Design review of the part built by this model. Coordinates are the model's own, in mm. A direction names the side the tool comes from. Round coordinates to 2 decimals unless told otherwise and drop trailing zeros. Loops run counter-clockwise (first coordinate to the right, second up) from the corner with the lowest first, then second, coordinate; pieces in that order, holes last. Notation, with made-up numbers: (42, -13.5) - (86, -13.5) arc R23 ccw to (86, 21.5) - close; hole circle Ø2 at (-6.75, 42.5). An arc over 180 degrees is marked (long way). Answer as CSV lines item,"result". Start each with the question number.
(1) Consider section A-A (y = -20). Give the boundary of the cut face in (x, z), and give its area (3 significant figures).
(2) For faces 4 (the cylindrical face through (-26.09, -81.57, -22.99)), 5 (the cylindrical face through (-23.92, 5.83, 27.37)), 6 (the flat face through (-23, 0, 22)), 7 (the flat face through (28, 6, -28)), list the 3-axis set-ups (+Z, -Z, +X, -X, +Y, -Y) from which the entire face can be reached by the end or side of a thin tool; tool diameter is ignored.
(3) For P1, Ø3, axis at x = 10.5, z = 14.5, coming from the +Y side; P2, Ø4.5, axis at x = -23.55, z = -23.55, coming from the +Y side; P3, Ø17.5, axis at x = 6, y = -75.5, coming from the +Z side; P4, Ø12, axis at x = 5.5, y = -17.5, coming from the +Z side, all flat-tipped, find the tip position at first contact; note any pin that passes through.
(4) Wall thickness on L1, parallel to X at y = -79, z = -23; L2, parallel to X at y = -69.5, z = 0; L3, parallel to Y at x = -20, z = 20.5: over which ranges is each line inside the solid? List them lowest first.
(5) Mouldability with a two-part tool opening along Y and no side actions: class faces 1 (the cylindrical face through (29.384, -27.98, 6.525)), 2 (the flat face through (24, -76.5, 24)), 3 (the flat face through (30, -75, 0)) as released by +Y, released by -Y, zero draft, split by the parting line, or undercut.
from build123d import *

# Parameters (mm, degrees)
IZIM1_W                      = 60
IZIM1_H                      = 60
Y_KSEKLIK_EKSTR_ZYON1_DEPTH  = 11.5
PAH1_SIZE                    = 4
IZIM2_R                      = 25
Y_KSEKLIK_EKSTR_ZYON2_DEPTH  = 3
PAH2_SIZE                    = 1
RADYUS1_R                    = 2
IZIM3_R                      = 30
Y_KSEKLIK_EKSTR_ZYON3_DEPTH  = 64.5
IZIM4_W                      = 60
IZIM4_H                      = 60
Y_KSEKLIK_EKSTR_ZYON4_DEPTH  = 22
PAH3_SIZE                    = 3
IZIM19_R                     = 8.5
Y_KSEKLIK_EKSTR_ZYON12_DEPTH = 2
IZIM20_R                     = 7
Y_KSEKLIK_EKSTR_ZYON13_DEPTH = 30
IZIM22_R                     = 2.75
KES_EKSTR_ZYON2_DEPTH        = 11.5
IZIM23_W                     = 0.1
IZIM23_H                     = 38.5
IZIM25_R                     = 2.6
KES_EKSTR_ZYON4_DEPTH        = 10


with BuildPart() as part:
    # Çizim1 → Yükseklik-Ekstrüzyon1 (new body)
    with BuildSketch(Plane(origin=(0, 0, 0), x_dir=(1, 0, 0), z_dir=(0, 1, 0))):
        Rectangle(IZIM1_W, IZIM1_H)
    extrude(amount=Y_KSEKLIK_EKSTR_ZYON1_DEPTH)

    # Pah1
    pah1_edges = [part.edges().sort_by_distance(p)[0] for p in [
        (30, 5.75, 30),
        (-30, 5.75, 30),
        (-30, 5.75, -30),
        (30, 5.75, -30),
    ]]
    chamfer(pah1_edges, length=PAH1_SIZE)

    # Çizim2 → Yükseklik-Ekstrüzyon2 (add)
    with BuildSketch(Plane(origin=(0, 11.5, 0), x_dir=(1, 0, 0), z_dir=(0, 1, 0))):
        with Locations(Location((0, 0, 0), (0, 0, 270))):
            Circle(IZIM2_R)
    extrude(amount=Y_KSEKLIK_EKSTR_ZYON2_DEPTH)

    # Pah2
    pah2_edges = [part.edges().sort_by_distance(p)[0] for p in [
        (0, 14.5, -25),
    ]]
    chamfer(pah2_edges, length=PAH2_SIZE)

    # Radyus1
    radyus1_edges = [part.edges().sort_by_distance(p)[0] for p in [
        (-30, 5.75, 26),
        (-30, 5.75, -26),
        (26, 5.75, -30),
        (-26, 5.75, -30),
        (26, 5.75, 30),
        (-26, 5.75, 30),
        (30, 5.75, 26),
        (30, 5.75, -26),
    ]]
    fillet(radyus1_edges, radius=RADYUS1_R)

    # Çizim3 → Yükseklik-Ekstrüzyon3 (add)
    with BuildSketch(Plane.XZ):
        with Locations(Location((0, 0, 0), (0, 0, 270))):
            Circle(IZIM3_R)
    extrude(amount=Y_KSEKLIK_EKSTR_ZYON3_DEPTH)

    # Çizim4 → Yükseklik-Ekstrüzyon4 (add)
    with BuildSketch(Plane.XZ.offset(64.5)):
        Rectangle(IZIM4_W, IZIM4_H)
    extrude(amount=Y_KSEKLIK_EKSTR_ZYON4_DEPTH)

    # Pah3
    pah3_edges = [part.edges().sort_by_distance(p)[0] for p in [
        (30, -75.5, -30),
        (30, -75.5, 30),
        (-30, -75.5, 30),
        (-30, -75.5, -30),
    ]]
    chamfer(pah3_edges, length=PAH3_SIZE)

    # Çizim8 → Kes-Döndür2 (revolve, cut)
    with BuildSketch(Plane(origin=(0, 0, 0), x_dir=(0, 0, -1), z_dir=(1, 0, 0))):
        with BuildLine():
            Line((-30, -64.5), (-40.4, -64.5))
            Line((-40.4, -64.5), (-40.4, -69.5))
            ThreePointArc((-40.4, -69.5), (-35.769748695, -65.814922715), (-30, -64.5))
        make_face()
    revolve(axis=Axis((0, -86.5, 0), (0, 1, 0)), mode=Mode.SUBTRACT)

    # Çizim19 → Yükseklik-Ekstrüzyon12 (add)
    with BuildSketch(Plane(origin=(0, 14.5, 0), x_dir=(1, 0, 0), z_dir=(0, 1, 0))):
        with Locations(Location((0, 0, 0), (0, 0, 270))):
            Circle(IZIM19_R)
    extrude(amount=Y_KSEKLIK_EKSTR_ZYON12_DEPTH)

    # Çizim20 → Yükseklik-Ekstrüzyon13 (add)
    with BuildSketch(Plane(origin=(0, 16.5, 0), x_dir=(1, 0, 0), z_dir=(0, 1, 0))):
        with Locations(Location((0, 0, 0), (0, 0, 270))):
            Circle(IZIM20_R)
    extrude(amount=Y_KSEKLIK_EKSTR_ZYON13_DEPTH)

    # Çizim22 → Kes-Ekstrüzyon2 (cut)
    with BuildSketch(Plane(origin=(0, 11.5, 0), x_dir=(1, 0, 0), z_dir=(0, 1, 0))):
        with Locations(Location((-24.748737342, 24.748737342, 0), (0, 0, 270))):
            Circle(IZIM22_R)
        with Locations(Location((24.748737342, 24.748737342, 0), (0, 0, 270))):
            Circle(IZIM22_R)
        with Locations(Location((24.748737342, -24.748737342, 0), (0, 0, 270))):
            Circle(IZIM22_R)
        with Locations(Location((-24.748737342, -24.748737342, 0), (0, 0, 270))):
            Circle(IZIM22_R)
    extrude(amount=-KES_EKSTR_ZYON2_DEPTH, mode=Mode.SUBTRACT)

    # Çizim23 → Döndür1 (revolve)
    with BuildSketch(Plane.XY, mode=Mode.PRIVATE) as d_nd_r1_sk:
        with Locations((-30.05, -28.25)):
            Rectangle(IZIM23_W, IZIM23_H)
    revolve(d_nd_r1_sk.sketch.rotate(Axis((0, -64.5, 0), (0, 1, 0)), 270), axis=Axis((0, -64.5, 0), (0, 1, 0)))

    # Çizim25 → Kes-Ekstrüzyon4 (cut)
    with BuildSketch(Plane(origin=(0, -86.5, 0), x_dir=(-1, 0, 0), z_dir=(0, -1, 0))):
        with Locations(Location((23.55, -23.55, 0), (0, 0, 90))):
            Circle(IZIM25_R)
        with Locations(Location((-23.55, -23.55, 0), (0, 0, 90))):
            Circle(IZIM25_R)
        with Locations(Location((23.55, 23.55, 0), (0, 0, 90))):
            Circle(IZIM25_R)
        with Locations(Location((-23.55, 23.55, 0), (0, 0, 90))):
            Circle(IZIM25_R)
    extrude(amount=-KES_EKSTR_ZYON4_DEPTH, mode=Mode.SUBTRACT)


solid = part.part
Determined:
1,outline,"circle Ø60.2 at (0, 0)"
1,area,"2,850 mm^2"
2,face 4,"-Y"
2,face 5,"+Y"
2,face 6,"+Z, -X"
2,face 7,"-Z, +X, +Y"
3,P1,"stops at y = 14.5"
3,P2,"stops at y = 11.5"
3,P3,"stops at z = 30"
3,P4,"stops at z = 30.1"
4,L1,"x = -30 to -26.09, -21.01 to 21.01, 26.09 to 30"
4,L2,"x = -30 to 30"
4,L3,"y = -86.5 to 11.5"
5,face 1,"undercut"
5,face 2,"released by -Y"
5,face 3,"zero draft"
